from build123d import *

# Parameters (mm, degrees)
F0_R     = 9
F1_DEPTH = 3.5
F2_DEPTH = 1
F0_R_2   = 6.25
F0_R_3   = 4
F3_DEPTH = 6.8
F4_DEPTH = 3


with BuildPart() as f1:
    # F0 (on Top) → F1 (new body)
    with BuildSketch(Plane.XY):
        with BuildLine():
            ThreePointArc((-8.752417, -27.042474), (-8.080641, -28.264092), (-6.773918, -28.75))
            Line((-6.773918, -28.75), (6.773918, -28.75))
            ThreePointArc((6.773918, -28.75), (8.080641, -28.264092), (8.752417, -27.042474))
            Line((8.752417, -27.042474), (12.75, 0))
            Line((12.75, 0), (12.75, 16.25))
            ThreePointArc((12.75, 16.25), (0, 28.75), (-12.75, 16.25))
            Line((-12.75, 16.25), (-12.75, 0))
            Line((-12.75, 0), (-8.752417, -27.042474))
        make_face()
        with BuildLine():
            Line((-4.75, -21.5), (-4.75, -12))
            ThreePointArc((-4.75, -12), (0, -7.25), (4.75, -12))
            Line((4.75, -12), (4.75, -21.5))
            ThreePointArc((4.75, -21.5), (0, -26.25), (-4.75, -21.5))
        make_face(mode=Mode.SUBTRACT)
        with Locations((0, 16.25)):
            Circle(F0_R, mode=Mode.SUBTRACT)
    extrude(amount=F1_DEPTH)

    # F0 (on Top) → F2 (join)
    with BuildSketch(Plane.XY):
        with BuildLine():
            ThreePointArc((-3, -15.68273), (-4.290251, -14.038688), (-4.75, -12))
            Line((-4.75, -12), (-4.75, -21.5))
            ThreePointArc((-4.75, -21.5), (0, -26.25), (4.75, -21.5))
            Line((4.75, -21.5), (4.75, -12))
            ThreePointArc((4.75, -12), (4.290251, -14.038688), (3, -15.68273))
            Line((3, -15.68273), (3, -21.5))
            ThreePointArc((3, -21.5), (0, -24.5), (-3, -21.5))
            Line((-3, -21.5), (-3, -15.68273))
        make_face()
    extrude(amount=F2_DEPTH)

    # F0 (on Top) → F3 (join)
    with BuildSketch(Plane.XY):
        with Locations((0, 16.25)):
            Circle(F0_R)
        with Locations((0, 16.25)):
            Circle(F0_R_2, mode=Mode.SUBTRACT)
        with Locations((0, 16.25)):
            Circle(F0_R_2)
        with Locations((0, 16.25)):
            Circle(F0_R_3, mode=Mode.SUBTRACT)
    extrude(amount=F3_DEPTH)

    # F0 (on Top) → F4 (cut)
    with BuildSketch(Plane.XY):
        with Locations((0, 16.25)):
            Circle(F0_R_2)
        with Locations((0, 16.25)):
            Circle(F0_R_3, mode=Mode.SUBTRACT)
    extrude(amount=F4_DEPTH, mode=Mode.SUBTRACT)


solid = f1.part
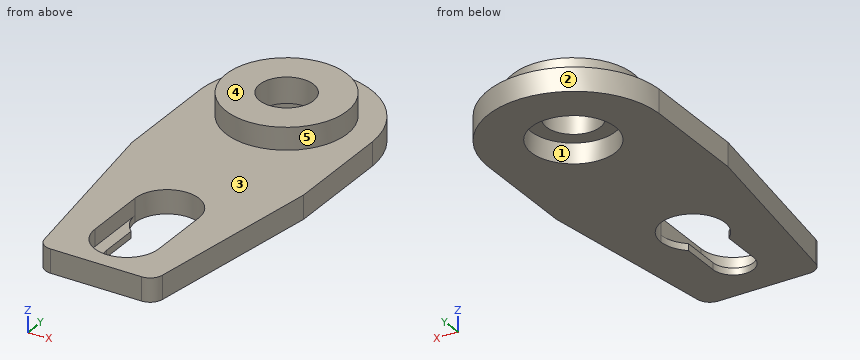
Check sheet for the modelled part. Datum: model origin and axes. Units: mm. Face numbers are marked on the shaded views. A direction names the side the tool comes from. Give positions to 0.01 mm unless a question says otherwise; leave off trailing zeros. Order: outer loops, then holes, each group sorted by start corner. A loop starts at its lowest first (then second) coordinate and runs counter-clockwise, first axis right, second up. Notation, with made-up numbers: (-30, 43) - (-25, 43) arc R27 cw to (-25, 65) - close; hole circle Ø7 at (54, 16). An arc over 180 degrees is marked (long way). Answer as CSV lines item,"result".
1. Scan lines: probe 1 along Y at (x, z) = (0, 2.15); probe 2 along Y at (x, z) = (0, 0.8); probe 3 along Y at (x, z) = (0, 4.95). Record each from-to range of solid material in increasing order. Write a range as from..to.
Result sheet:
probe 1,"-28.75..-26.25, -7.25..10, 22.5..28.75"
probe 2,"-28.75..-24.5, -7.25..10, 22.5..28.75"
probe 3,"7.25..12.25, 20.25..25.25"
2. Section check D-D (y = 1). Record the boundary of the cut face in (x, z), then the cut area to 4 significant figures.
Result sheet:
outline,"(-12.75, 0) - (12.75, 0) - (12.75, 3.5) - (-12.75, 3.5) - close"
area,"89.25 mm²"
3. Section check B-B (z = 2). State how many separate pieces and enclosed holes the cut face has, then the cut area to 3 significant figures.
Result sheet:
separate pieces,"1"
enclosed holes,"2"
area,"989 mm²"
4. Tool access check on the marked faces 4 and 5. Record the directions out of +Z, -Z, +X, -X, +Y, -Y that give a thin tool (end or side, any length) a straight path to the whole face; none if there is none.
Result sheet:
face 4,"+Z, +X, -X, +Y, -Y"
face 5,"+Z"
5. Section check A-A (x = 0). Record the boundary of the cut face in (y, z), then the cut area to 3 significant figures.
Result sheet:
outline,"(-28.75, 0) - (-24.5, 0) - (-24.5, 1) - (-26.25, 1) - (-26.25, 3.5) - (-28.75, 3.5) - close; (-7.25, 0) - (10, 0) - (10, 3) - (12.25, 3) - (12.25, 6.8) - (7.25, 6.8) - (7.25, 3.5) - (-7.25, 3.5) - close; (20.25, 3) - (22.5, 3) - (22.5, 0) - (28.75, 0) - (28.75, 3.5) - (25.25, 3.5) - (25.25, 6.8) - (20.25, 6.8) - close"
area,"128 mm²"
6. Section check C-C (y = 18.5). Record the boundary of the cut face in (x, z), then the cut area to 3 significant figures.
Result sheet:
outline,"(-12.5, 0) - (-5.83, 0) - (-5.83, 3) - (-3.31, 3) - (-3.31, 6.8) - (-8.71, 6.8) - (-8.71, 3.5) - (-12.5, 3.5) - close; (3.31, 3) - (5.83, 3) - (5.83, 0) - (12.5, 0) - (12.5, 3.5) - (8.71, 3.5) - (8.71, 6.8) - (3.31, 6.8) - close"
area,"84.9 mm²"
7. Mould release check, pull along Y, two halves, no side actions. Record for the marked faces 1, 2 and 3: released by +Y, released by -Y, zero draft, split by the parting line, or undercut.
Result sheet:
face 1,"undercut"
face 2,"released by +Y"
face 3,"zero draft"
8. Go/stop test with flat-tipped pins: P1, Ø10, axis at x = 5.5, y = -16.5, coming from the +Z side; P2, Ø2, axis at y = -18, z = 2, coming from the +X side; P3, Ø1.1, axis at y = -18, z = 0.5, coming from the -X side. Record where each tip stops, or that it passes through.
Result sheet:
P1,"z = 3.5"
P2,"x = 10.24"
P3,"x = -10.17"
